Autodesk Inventor part; units mm, degrees
ref_plane "YZ Plane" through (0, 0, 0) normal (1, 0, 0) x (0, 1, 0)
ref_plane "XZ Plane" through (0, 0, 0) normal (0, 1, 0) x (-1, 0, 0)
ref_plane "XY Plane" through (0, 0, 0) normal (0, 0, 1) x (1, 0, 0)
sketch "Sketch1" plane through (0, 0, 0) normal (0, 0, 1) x (1, 0, 0)
  circle A0 centre (0, 0) radius 22.5
  circle A1 centre (0, 0) radius 17.5
  line L0 (0, 0) -> (0, 22.5)
  line L1 (0, 22.5) -> (0, 0)
  line L2 (6.9529, 21.3988) -> (0, 0)
  line L3 (0, 0) -> (2.7376, 17.2845)
  line L4 (0, 22.5) -> (2.7376, 17.2845)
  line L5 (6.9529, 21.3988) -> (2.7376, 17.2845)
  line L6 (-6.9529, 21.3988) -> (-2.7376, 17.2845)
  line L7 (0, 22.5) -> (-2.7376, 17.2845)
  line L8 (-13.2252, 18.2029) -> (-7.9448, 15.5926)
  line L9 (-6.9529, 21.3988) -> (-7.9448, 15.5926)
  line L10 (-18.2029, 13.2252) -> (-12.3744, 12.3744)
  line L11 (-13.2252, 18.2029) -> (-12.3744, 12.3744)
  line L12 (-21.3988, 6.9529) -> (-15.5926, 7.9448)
  line L13 (-18.2029, 13.2252) -> (-15.5926, 7.9448)
  line L14 (-22.5, 0) -> (-17.2845, 2.7376)
  line L15 (-21.3988, 6.9529) -> (-17.2845, 2.7376)
  line L16 (-21.3988, -6.9529) -> (-17.2845, -2.7376)
  line L17 (-22.5, 0) -> (-17.2845, -2.7376)
  line L18 (-18.2029, -13.2252) -> (-15.5926, -7.9448)
  line L19 (-21.3988, -6.9529) -> (-15.5926, -7.9448)
  line L20 (-13.2252, -18.2029) -> (-12.3744, -12.3744)
  line L21 (-18.2029, -13.2252) -> (-12.3744, -12.3744)
  line L22 (-6.9529, -21.3988) -> (-7.9448, -15.5926)
  line L23 (-13.2252, -18.2029) -> (-7.9448, -15.5926)
  line L24 (0, -22.5) -> (-2.7376, -17.2845)
  line L25 (-6.9529, -21.3988) -> (-2.7376, -17.2845)
  line L26 (6.9529, -21.3988) -> (2.7376, -17.2845)
  line L27 (0, -22.5) -> (2.7376, -17.2845)
  line L28 (13.2252, -18.2029) -> (7.9448, -15.5926)
  line L29 (6.9529, -21.3988) -> (7.9448, -15.5926)
  line L30 (18.2029, -13.2252) -> (12.3744, -12.3744)
  line L31 (13.2252, -18.2029) -> (12.3744, -12.3744)
  line L32 (21.3988, -6.9529) -> (15.5926, -7.9448)
  line L33 (18.2029, -13.2252) -> (15.5926, -7.9448)
  line L34 (22.5, 0) -> (17.2845, -2.7376)
  line L35 (21.3988, -6.9529) -> (17.2845, -2.7376)
  line L36 (21.3988, 6.9529) -> (17.2845, 2.7376)
  line L37 (22.5, 0) -> (17.2845, 2.7376)
  line L38 (18.2029, 13.2252) -> (15.5926, 7.9448)
  line L39 (21.3988, 6.9529) -> (15.5926, 7.9448)
  line L40 (13.2252, 18.2029) -> (12.3744, 12.3744)
  line L41 (18.2029, 13.2252) -> (12.3744, 12.3744)
  line L42 (6.9529, 21.3988) -> (7.9448, 15.5926)
  line L43 (13.2252, 18.2029) -> (7.9448, 15.5926)
  point P0 (-22.5, 0)
  point P1 (-6.9529, -21.3988)
  point P2 (0, -22.5)
  point P3 (6.9529, -21.3988)
  point P4 (13.2252, -18.2029)
  point P5 (18.2029, -13.2252)
  point P6 (21.3988, -6.9529)
  point P7 (22.5, 0)
  point P8 (21.3988, 6.9529)
  point P9 (18.2029, 13.2252)
  point P10 (15.5926, 7.9448)
  point P11 (12.3744, 12.3744)
  point P12 (7.9448, 15.5926)
  point P13 (-21.3988, 6.9529)
  point P14 (-22.5, 0)
  point P15 (-21.3988, -6.9529)
  point P16 (-18.2029, -13.2252)
  point P17 (-13.2252, -18.2029)
  point P18 (-6.9529, -21.3988)
  point P19 (0, -22.5)
  point P20 (6.9529, -21.3988)
  point P21 (13.2252, -18.2029)
  point P22 (22.5, 0)
  point P23 (18.2029, 13.2252)
  point P24 (13.2252, 18.2029)
  dimension "d4" = 45
  dimension "d28" = 5
  dimension "d2" = 360
  dimension "d6" = 18
  dimension "d7" = 9
  dimension "d10" = 360
  dimension "d14" = 360
extrude "Extrusion1" add sketch "Sketch1" along normal blind 5 contours L34 A1 L37 | L36 A1 L39 | L32 A1 L35 | A1 L0 L2 | L38 A1 L41 | L30 A1 L33 | L40 A1 L43 | L28 A1 L31 | L42 A1 L2 | L2 A1 L5 | L26 A1 L29 | L4 A1 L0 | L0 A1 L7 | L2 L3 A1 | L3 L0 A1 | L24 A1 L27 | L6 A1 L9 | L22 A1 L25 | L8 A1 L11 | L20 A1 L23 | L10 A1 L13 | L18 A1 L21 | L12 A1 L15 | L16 A1 L19 | L14 A1 L17
sketch "Sketch2" plane through (0, 0, 0) normal (0, 0, -1) x (-1, 0, 0)
  line L0 (-2.7376, 17.2845) -> (0, 22.5)
  circle A0 centre (0, 0) radius 22.5
  circle A1 centre (0, 0) radius 21.8
  dimension "d18" = 0.7
extrude "Extrusion2" cut sketch "Sketch2" against normal blind 5
sketch "Sketch3" plane through (0, 0, 0) normal (0, 0, -1) x (-1, 0, 0)
  point P0 (0, 0)
hole "Hole1" at (0, 0, 0) direction (0, 0, 1) diameter 4.134 depth 14.2 tip angle 118
properties part number "Gear_Basic"
CAD build for the part. Positions are in the model's coordinates, mm. A direction names the side the tool comes from. Round coordinates to 2 decimals unless told otherwise and drop trailing zeros. Loops run counter-clockwise (first coordinate to the right, second up) from the corner with the lowest first, then second, coordinate; pieces in that order, holes last.
(1) Cut at B-B (x = -9). Give the cut face in (y, z), plus the area to 3 significant figures.
(2) Wall check: line 1 along Y through (x, z) = (-16.5, 0.8); line 2 along X through (y, z) = (-17, 1.5); line 3 along X through (y, z) = (0, 3.95). Give the ranges that are in metal, low to high.
(3) Which spindle directions (+Z, -Z, +X, -X, +Y, -Y) get a long thin tool onto all of the face, cutting with end or side? Do faces 1 (the flat face through (0, -5, 0)), 2 (the flat face through (10.261, 16.738, 2.465)), 3 (the flat face through (19.1, 4.6, 2.5)), 4 (the flat face through (-16.738, -10.261, 2.465)), 5 (the flat face through (-1.54, -19.57, 2.46)). Say none if no direction does.
(4) Drop flat-ended pins along their axis: pin 1 (1.5 mm diameter, centred on y = -6.5, z = 3.5, fed in from +X); pin 2 (1.5 mm diameter, centred on y = 9.5, z = 1, fed in from +X); pin 3 (3 mm diameter, centred on x = -12, z = 4, fed in from +Y). Give the stop position or say it passes through.
(5) Two-plate mould, pull along X, no slides. Class faces 6 (the flat face through (16.738, 10.261, 2.465)), 7 (the flat face through (-19.1, 4.6, 2.5)), 8 (the flat face through (-14.931, -12.748, 2.465)): +X half, -X half, draft (parallel to the pull), parting line (faces both ways), or undercut.
(6) Cut at C-C (y = 5.5). Give the cut face in (x, z), plus the area to 3 significant figures.
(7) Cut at A-A (x = -1.5). Give the cut face in (y, z).
Findings below:
1. outline: (-16.11, 0) - (16.11, 0) - (16.11, 5) - (-16.11, 5) - close
1. area: 161 mm2
2. line 1: y = -12.98 to -9.78, -7.79 to 7.79, 9.78 to 12.98
2. line 2: x = -13.05 to -10.79, -7.7 to 7.7, 10.79 to 13.05
2. line 3: x = -21.8 to -2.07, 2.07 to 21.8
3. face 1: -Z, +X, -X, +Y, -Y
3. face 2: +Z, -Z, +Y
3. face 3: +Z, -Z, +X
3. face 4: +Z, -Z, -X
3. face 5: +Z, -Z, -Y
4. pin 1: stops at x = 20.84
4. pin 2: stops at x = 16.73
4. pin 3: stops at y = 17.85
5. face 6: +X half
5. face 7: -X half
5. face 8: undercut
6. outline: (-19.98, 0) - (19.98, 0) - (19.98, 5) - (-19.98, 5) - close
6. area: 200 mm2
7. outline: (-19.64, 0) - (-1.42, 0) - (-1.42, 5) - (-19.64, 5) - close; (1.42, 0) - (19.64, 0) - (19.64, 5) - (1.42, 5) - close
